Autodesk Inventor part; units mm, degrees
ref_plane "XZ Plane" through (0, 0, 0) normal (0, 1, 0) x (-1, 0, 0)
ref_plane "XY Plane" through (0, 0, 0) normal (0, 0, 1) x (1, 0, 0)
sketch "스케치1" plane through (0, 0, 0) normal (0, 0, 1) x (1, 0, 0)
  line L0 (0, 0) -> (-10, 0)
  line L1 (-10, 0) -> (-10, -15)
  line L2 (-10, -15) -> (-3.5, -15)
  line L3 (-3.5, -15) -> (-3.5, -25)
  line L4 (-3.5, -25) -> (-7.5, -25)
  line L5 (-7.5, -25) -> (-7.5, -30)
  line L6 (-7.5, -30) -> (0, -30)
  line L7 (0, 0) -> (0, -30)
  dimension "d0" = 10
  dimension "d1" = 15
  dimension "d2" = 10
  dimension "d3" = 5
  dimension "d4" = 7.5
  dimension "d12" = 3.5
extrude "돌출1" add sketch "스케치1" along normal mid plane 8
mirror "미러1" about plane through (0, 0, 0) normal (1, 0, 0) of "돌출1"
fillet "모깎기1" radius 5 2 edges at (10, 0, 0) (-10, 0, 0)
sketch "스케치2" plane through (0, 0, 4) normal (0, 0, 1) x (1, 0, 0)
  line L0 (-6.452, -3.1686) -> (7.8296, -3.1686) construction
  line L1 (7.8296, -3.1686) -> (7.8296, -13.9142) construction
  line L2 (7.8296, -13.9142) -> (-6.452, -13.9142) construction
  line L3 (-6.452, -13.9142) -> (-6.452, -3.1686) construction
  line L4 (0.4443, -13.3793) -> (-5.7226, -13.3793)
  line L5 (-5.7226, -13.3793) -> (-5.7226, -11.9611)
  spline S0 degree 2 poles (-5.7226, -11.9611) (-5.0581, -11.3371) (-3.875, -10.1783) (-3.3077, -9.5543) knots 0 0 0 1 2 2 2
  spline S1 degree 2 poles (-3.3077, -9.5543) (-2.1651, -8.2982) (-1.3304, -6.7909) (-1.3304, -5.9887) knots 0 0 0 1 2 2 2
  spline S2 degree 2 poles (-1.3304, -5.9887) (-1.3304, -5.5673) (-1.5897, -4.9352) (-1.8247, -4.7326) knots 0 0 0 1 2 2 2
  spline S3 degree 2 poles (-1.8247, -4.7326) (-2.0597, -4.53) (-2.6756, -4.3274) (-3.0484, -4.3274) knots 0 0 0 1 2 2 2
  spline S4 degree 2 poles (-3.0484, -4.3274) (-3.405, -4.3274) (-4.1343, -4.5057) (-4.4665, -4.6435) knots 0 0 0 1 2 2 2
  spline S5 degree 2 poles (-4.4665, -4.6435) (-4.7502, -4.7569) (-5.2769, -5.0811) (-5.439, -5.1945) knots 0 0 0 1 2 2 2
  line L6 (-5.439, -5.1945) -> (-5.5119, -5.1945)
  line L7 (-5.5119, -5.1945) -> (-5.5119, -3.7683)
  spline S6 degree 2 poles (-5.5119, -3.7683) (-5.0986, -3.5657) (-3.6157, -3.1686) (-2.9511, -3.1686) knots 0 0 0 1 2 2 2
  spline S7 degree 2 poles (-2.9511, -3.1686) (-1.5492, -3.1686) (0.031, -4.6516) (0.031, -5.9157) knots 0 0 0 1 2 2 2
  spline S8 degree 2 poles (0.031, -5.9157) (0.031, -6.5073) (-0.2445, -7.496) (-0.4876, -7.9174) knots 0 0 0 1 2 2 2
  spline S9 degree 2 poles (-0.4876, -7.9174) (-0.7307, -8.355) (-1.4358, -9.214) (-1.8247, -9.6272) knots 0 0 0 1 2 2 2
  spline S10 degree 2 poles (-1.8247, -9.6272) (-2.4568, -10.3161) (-4.0046, -11.7909) (-4.4665, -12.2204) knots 0 0 0 1 2 2 2
  line L8 (-4.4665, -12.2204) -> (0.4443, -12.2204)
  line L9 (0.4443, -12.2204) -> (0.4443, -13.3793)
  line L10 (7.4459, -13.3793) -> (2.5675, -13.3793)
  line L11 (2.5675, -13.3793) -> (2.5675, -12.3582)
  line L12 (2.5675, -12.3582) -> (4.3827, -12.3582)
  line L13 (4.3827, -12.3582) -> (4.3827, -5.6564)
  line L14 (4.3827, -5.6564) -> (2.5675, -5.6564)
  line L15 (2.5675, -5.6564) -> (2.5675, -4.7407)
  spline S11 degree 2 poles (2.5675, -4.7407) (3.5967, -4.7407) (4.5691, -4.1572) (4.6339, -3.3469) knots 0 0 0 1 2 2 2
  line L16 (4.6339, -3.3469) -> (5.6712, -3.3469)
  line L17 (5.6712, -3.3469) -> (5.6712, -12.3582)
  line L18 (5.6712, -12.3582) -> (7.4459, -12.3582)
  line L19 (7.4459, -12.3582) -> (7.4459, -13.3793)
  point P0 (0, 0)
extrude "돌출2" cut sketch "스케치2" against normal blind 1
properties part number "2번부품"
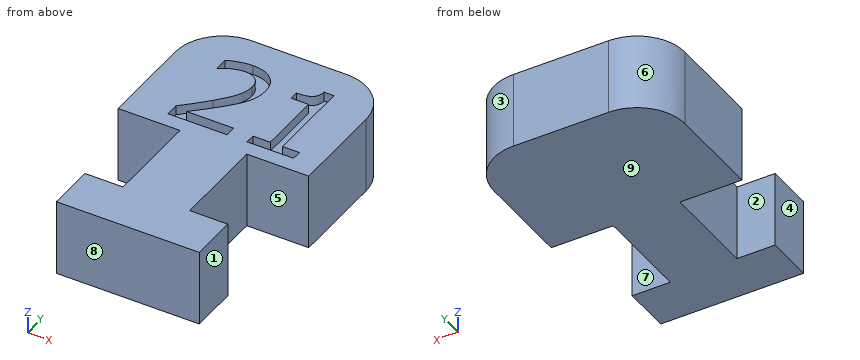
Here's how the part is built. I have some questions about the finished solid (model axes, mm). Face numbers are marked on the shaded views. A direction names the side the tool comes from. Coordinates: 2 decimals unless noted, no trailing zeros. Loops run counter-clockwise (first coordinate to the right, second up) from the corner with the lowest first, then second, coordinate; pieces in that order, holes last.
1. For the marked faces 1, 2, 3, 4 and 5, which set-ups out of +Z, -Z, +X, -X, +Y, -Y let a thin tool reach every point of the face, with its end or its side?
2. I need wall thicknesses on L1, parallel to Y at x = -4, z = 1.25; L2, parallel to X at y = -20.5, z = 3.5; L3, parallel to Y at x = -0.5, z = 3.5. Which ranges of each line are inside material? Lowest first, please.
3. Imagine slicing it at D-D, the plane x = -8. Please give me the cut outline in (y, z), and give its area (3 significant figures).
4. For P1, Ø1.5, axis at y = -28, z = 2, coming from the -X side; P2, Ø4, axis at y = -28.5, z = -1, coming from the +X side, each with a flat end and sliding along its axis, tell me the tip position at first contact or that it passes through.
5. Imagine slicing it at B-B, the plane x = 6.25. Please give me the cut outline in (y, z).
6. Imagine slicing it at C-C, the plane y = -13. Please give me the cut outline in (x, z).
7. Imagine slicing it at A-A, the plane z = 1.75. Please give me the cut outline in (x, y), and give its area (3 significant figures).
8. If we mould it in two halves opening along Y, with no side actions, what happens to the marked faces 6, 7, 8 and 9? For each: pulls with the +Y half, pulls with the -Y half, needs draft (parallel to the pull), parting line crosses it, or undercut.
Taken from the geometry:
1. face 1: +Z, -Z, +X, -Y
1. face 2: +Z, -Z, -X
1. face 3: +Z, -Z, +X, +Y
1. face 4: +Z, -Z, -X, -Y
1. face 5: +Z, -Z, +X
2. L1: y = -30 to -25, -15 to 0
2. L2: x = -3.5 to 3.5
2. L3: y = -30 to -13.38, -12.22 to -7.94, -4.19 to 0
3. outline: (-15, -4) - (-1, -4) - (-1, 4) - (-15, 4) - close
3. area: 112 mm2
4. P1: stops at x = -7.5
4. P2: stops at x = 7.5
5. outline: (-30, -4) - (-25, -4) - (-25, 4) - (-30, 4) - close; (-15, -4) - (-0.16, -4) - (-0.16, 4) - (-12.36, 4) - (-12.36, 3) - (-13.38, 3) - (-13.38, 4) - (-15, 4) - close
6. outline: (-10, -4) - (10, -4) - (10, 4) - (7.45, 4) - (7.45, 3) - (2.57, 3) - (2.57, 4) - (0.44, 4) - (0.44, 3) - (-5.72, 3) - (-5.72, 4) - (-10, 4) - close
7. outline: (-10, -15) - (-3.5, -15) - (-3.5, -25) - (-7.5, -25) - (-7.5, -30) - (7.5, -30) - (7.5, -25) - (3.5, -25) - (3.5, -15) - (10, -15) - (10, -5) arc R5 ccw to (5, 0) - (-5, 0) arc R5 ccw to (-10, -5) - close
7. area: 434 mm2
8. face 6: pulls with the +Y half
8. face 7: undercut
8. face 8: pulls with the -Y half
8. face 9: needs draft
